Model file for the job. Use its own axes, mm. A direction names the side the tool comes from. Round coordinates to 2 decimals unless told otherwise and drop trailing zeros. Loops run counter-clockwise (first coordinate to the right, second up) from the corner with the lowest first, then second, coordinate; pieces in that order, holes last. Notation, with made-up numbers: M -0.75,42 L 15.25,42 A16 ccw 15.25,63 Z; hole C 12.25,63 d8. An arc over 180 degrees is marked long. Use a Markdown table: item, result. Add a question column.
Item 1: Wall check: L1, parallel to X at y = -0.3, z = 28; L2, parallel to Z at x = -27.5, y = -1.35; L3, parallel to Z at x = -39, y = -0.85. Give the ranges that are in metal, low to high. Write a range as from..to.
Item 2: Saw through at A-A on z = 26.5. Write the cut outline in (x, y).
Item 3: Saw through at B-B on x = -40.5. Write the cut outline in (y, z), then the cut area to 3 significant figures.
Item 4: Saw through at C-C on z = -6. Write the cut outline in (x, y).
Item 5: Pin check, flat tips, straight feed: P1, Ø0.9, axis at x = 36.5, y = -1.5, coming from the +Z side; P2, Ø0.9, axis at x = 17.5, y = -2, coming from the +Z side; P3, Ø1, axis at x = 24, y = -2, coming from the -Z side. Stop position of each tip, or through.
Item 6: Two-plate mould, pull along X, no slides. Class faces 1 (the flat face through (-4.642, -1, 11)), 2 (the flat face through (-51.786, -1, 5)), 3 (the flat face through (3, -1, 15.789)): +X half, -X half, draft (parallel to the pull), parting line (faces both ways), or undercut.
Item 7: Tool access for faces 4 (the cylindrical face through (99.467, -1.479, 13.935)), 5 (the flat face through (-4.61, -1, -2)), 6 (the flat face through (-29, -1, 10)), 7 (the flat face through (49, 0, 2)), 8 (the flat face through (11.358, -1, 11)): list every direction of +Z, -Z, +X, -X, +Y, -Y with a clear straight run to the whole face (end or side of a thin tool).
```python
from build123d import *

# Parameters (mm, degrees)
F1_DEPTH = 3


with BuildPart() as f1:
    # F0 (on Front) → F1 (new body)
    with BuildSketch(Plane.XZ):
        with BuildLine():
            Line((-36.785731, 10), (-51.785731, 10))
            Line((-51.785731, 10), (-51.785731, 0))
            Line((-51.785731, 0), (-36.785731, 0))
            Line((-36.785731, 0), (-36.666999, 0))
            ThreePointArc((-36.666999, 0), (-28.666999, -4.433981), (-20.666999, 0))
            Line((-20.666999, 0), (-4.60982, -4.364454))
            Line((-4.60982, -4.364454), (-4.60982, 0))
            Line((-4.60982, 0), (78.480504, -11.91812))
            Line((78.480504, -11.91812), (91.646317, 2.007614))
            ThreePointArc((91.646317, 2.007614), (114.40079, 11.115801), (98.197224, 29.505187))
            ThreePointArc((98.197224, 29.505187), (99.359, 13.727695), (85.650786, 5.830618))
            ThreePointArc((85.650786, 5.830618), (85.195749, 5.854985), (84.741672, 5.893281))
            ThreePointArc((84.741672, 5.893281), (84.691969, 5.979948), (84.642764, 6.066899))
            ThreePointArc((84.642764, 6.066899), (79.456589, 9.015264), (76.264674, 14.055199))
            Line((76.264674, 14.055199), (64.344662, 35.789207))
            Line((64.344662, 35.789207), (50.344662, 35.789207))
            Line((50.344662, 35.789207), (50.344662, 5.789207))
            Line((50.344662, 5.789207), (47.344662, 5.789207))
            Line((47.344662, 5.789207), (47.344662, 15.789207))
            Line((47.344662, 15.789207), (37.358069, 15.789207))
            Line((37.358069, 15.789207), (37.358069, 5.789207))
            Line((37.358069, 5.789207), (34.358069, 5.789207))
            Line((34.358069, 5.789207), (34.358069, 15.789207))
            Line((34.358069, 15.789207), (24.358069, 15.789207))
            Line((24.358069, 15.789207), (24.358069, 5.789207))
            Line((24.358069, 5.789207), (21.358069, 5.789207))
            Line((21.358069, 5.789207), (21.358069, 15.789207))
            Line((21.358069, 15.789207), (11.358069, 15.789207))
            Line((11.358069, 15.789207), (11.358069, 5.789207))
            Line((11.358069, 5.789207), (8.358069, 5.789207))
            Line((8.358069, 5.789207), (8.358069, 15.789207))
            Line((8.358069, 15.789207), (-1.641931, 15.789207))
            Line((-1.641931, 15.789207), (-1.641931, 5.789207))
            Line((-1.641931, 5.789207), (-4.641931, 5.789207))
            Line((-4.641931, 5.789207), (-4.641931, 15.789207))
            Line((-4.641931, 15.789207), (-23.785731, 10))
            Line((-23.785731, 10), (-33.785731, 10))
            Line((-33.785731, 10), (-33.785731, 5))
            Line((-33.785731, 5), (-36.785731, 5))
            Line((-36.785731, 5), (-36.785731, 10))
        make_face()
    extrude(amount=F1_DEPTH)


solid = f1.part
```
Entries:
| question | item | result |
|---|---|---|
| 1 | L1 | 50.34..68.62, 99.17..106.53 |
| 1 | L2 | -4.36..10 |
| 1 | L3 | 0..10 |
| 2 | outline | M 50.34,-3 L 69.44,-3 L 69.44,0 L 50.34,0 Z; M 99.91,-3 L 108.93,-3 L 108.93,0 L 99.91,0 Z |
| 3 | outline | M -3,0 L 0,0 L 0,10 L -3,10 Z |
| 3 | area | 30.0 mm2 |
| 4 | outline | M 37.22,-3 L 84.08,-3 L 84.08,0 L 37.22,0 Z |
| 5 | P1 | z = 5.79 |
| 5 | P2 | z = 15.79 |
| 5 | P3 | z = -4.18 |
| 6 | face 1 | undercut |
| 6 | face 2 | -X half |
| 6 | face 3 | draft |
| 7 | face 4 | +Y, -Y |
| 7 | face 5 | -Z, +Y, -Y |
| 7 | face 6 | +Z, -X, +Y, -Y |
| 7 | face 7 | +Z, -Z, +X, -X, +Y |
| 7 | face 8 | +Z, +Y, -Y |
